The model under review builds one solid part; all positions refer to its coordinate system, in mm. A direction names the side the tool comes from. Give positions to 0.01 mm unless a question says otherwise; leave off trailing zeros. Order: outer loops, then holes, each group sorted by start corner. A loop starts at its lowest first (then second) coordinate and runs counter-clockwise, first axis right, second up. Notation, with made-up numbers: (69, 51) - (125, 51) arc R15 ccw to (125, 57) - close; hole circle Ø5 at (-18, 61.25). An arc over 180 degrees is marked (long way). Write item = value, one per line. Start each with the question number.
1. We need section C-C, the plane z = 3.5. Give the boundary of the cut face in (x, y), and give its area (3 significant figures).
2. Mouldability with a two-part tool opening along Z and no side actions: class faces 1 (the cylindrical face through (-7.815, 5.07, 1.243)), 2 (the conical face through (-0.038, -4.376, -1.747)), 3 (the cylindrical face through (3.727, 5.07, -7.095)), 4 (the cylindrical face through (-7.9, 5.07, -1.35)) as pulls with the +Z half, pulls with the -Z half, needs draft (parallel to the pull), parting line crosses it, or undercut.
3. We need section B-B, the plane x = 7. Give the boundary of the cut face in (y, z).
4. Wall thickness on probe 1 along Y at (x, z) = (2.5, 3.75); probe 2 along X at (y, z) = (7.25, 6); probe 3 along X at (y, z) = (9.5, -1.5): over which ranges is each line inside the solid? List them lowest first.
5. For P1, Ø1.1, axis at x = 0, z = -0.5, coming from the +Y side (3 decimals); P2, Ø3, axis at x = 4.5, y = 3, coming from the -Z side; P3, Ø1.5, axis at x = 4, y = -2.5, coming from the +Z side, all flat-tipped, find the tip position at first contact; note any pin that passes through.
6. Machinability: for faces 5 (the cylindrical face through (1.155, 5.07, 7.93)), 6 (the flat face through (0, 5, 2.2)), 7 (the flat face through (0, -5, 0)), which of the approach directions +Z, -Z, +X, -X, +Y, -Y give a long, thin tool a straight path to every point of the face, cutting with its end or side? Answer none if there is none.
from build123d import *
from build123d import SkipClean  # not in build123d's __all__

# Parameters (mm, degrees)
F0_W            = 6.5
F0_H            = 10
F3_DEPTH        = 25
F5_DEPTH        = 10
F5_COPIES_COUNT = 10
F7_DEPTH        = 6.5
F9_SIZE         = 2.5


# Not quite as in the source:
# - a pattern or mirror of a feature is missing from the dataset's text; its kind, count and spacing are read off the source's solid
# - a feature names something its author has since deleted; it is built from what else it names


with BuildPart() as f1:
    # F0 (on Top) → F1 (revolve)
    with BuildSketch(Plane.XY):
        with Locations((-3.25, 5)):
            Rectangle(F0_W, F0_H)
    revolve(axis=Axis((0, 5, 0), (0, 1, 0)))

    # F2 (on face) → F3 (cut)
    with BuildSketch(Plane(origin=(0, 10, 0), x_dir=(-1, 0, 0), z_dir=(0, 1, 0))):
        with BuildLine():
            Line((1.65, 2.2), (-1.65, 2.2))
            ThreePointArc((-1.65, 2.2), (0, -2.75), (1.65, 2.2))
        make_face()
    extrude(amount=-F3_DEPTH, mode=Mode.SUBTRACT)

    # F4 (on face) → F5 (join)
    with BuildSketch(Plane(origin=(0, 10, 0), x_dir=(-1, 0, 0), z_dir=(0, 1, 0))):
        with BuildLine():
            ThreePointArc((-2.0086104634, 6.1818673559), (0.0140777422, 6.4999847551), (2.0353690139, 6.1731088584))
            ThreePointArc((2.0353690139, 6.1731088584), (1.2263837508, 7.8268898276), (0, 9.2))
            ThreePointArc((0, 9.2), (-1.1693294851, 7.9103781541), (-1.9692767773, 6.3642409415))
            ThreePointArc((-1.9692767773, 6.3642409415), (-1.9898456325, 6.2732486915), (-2.0086104634, 6.1818673559))
        make_face()
    f5 = extrude(amount=-F5_DEPTH)

    # F5_copies: F5 ×10 about axis
    f5_copies_axis = Axis((0, 0, 0), (0, 1, 0))
    for i in range(1, F5_COPIES_COUNT):
        add(f5.rotate(f5_copies_axis, i * 360 / F5_COPIES_COUNT), clean=False)

    # F6 (on face) → F7 (join)
    with BuildSketch(Plane.XZ):
        with BuildLine():
            Line((-2.75, 0), (-4.75, 0))
            ThreePointArc((-4.75, 0), (0, -4.75), (4.75, 0))
            Line((4.75, 0), (2.75, 0))
            ThreePointArc((2.75, 0), (0, -2.75), (-2.75, 0))
        make_face()
        with BuildLine():
            Line((2.75, 0), (-2.75, 0))
            ThreePointArc((-2.75, 0), (0, -2.75), (2.75, 0))
        make_face()
    extrude(amount=F7_DEPTH)

    # F9
    f9_edges = [f1.edges().sort_by_distance(p)[0] for p in [
        (0, -6.5, -4.75),
    ]]
    chamfer(f9_edges, length=F9_SIZE)

    # F8 (on face) → F10 (revolve, cut)
    with BuildSketch(Plane.XY):
        Polygon((0, -1.3273195364), (0, 0), (-2.75, 0), (-2.75, -3.3025264561), (-1.375, -4.775), (0, -4.775), (0, -3.3025264561), (0, -1.8300529122), align=None)
    with SkipClean():  # cleaning this boolean's faces spoils the solid; the shape is the same uncleaned
        revolve(axis=Axis((0, -3.3025264561, 0), (0, -1, 0)), mode=Mode.SUBTRACT)


solid = f1.part
Model answer:
q1.outline = (-7.34, 0) - (7.34, 0) - (7.34, 10) - (-7.34, 10) - close
q1.area = 147 mm2
q2.face_1 = undercut
q2.face_2 = pulls with the +Z half
q2.face_3 = pulls with the -Z half
q2.face_4 = undercut
q3.outline = (0, -3.6) - (10, -3.6) - (10, -0.38) - (0, -0.38) - close; (0, 0.38) - (10, 0.38) - (10, 3.6) - (0, 3.6) - close
q4.probe_1 = 0 to 10
q4.probe_2 = -5.6 to 5.6
q4.probe_3 = -8.01 to -2.3, 2.3 to 8.01
q5.P1 = -4.775
q5.P2 = -7.44
q5.P3 = 0
q6.face_5 = +Z, +Y, -Y
q6.face_6 = +Y, -Y
q6.face_7 = +Z, +X, -X, -Y
